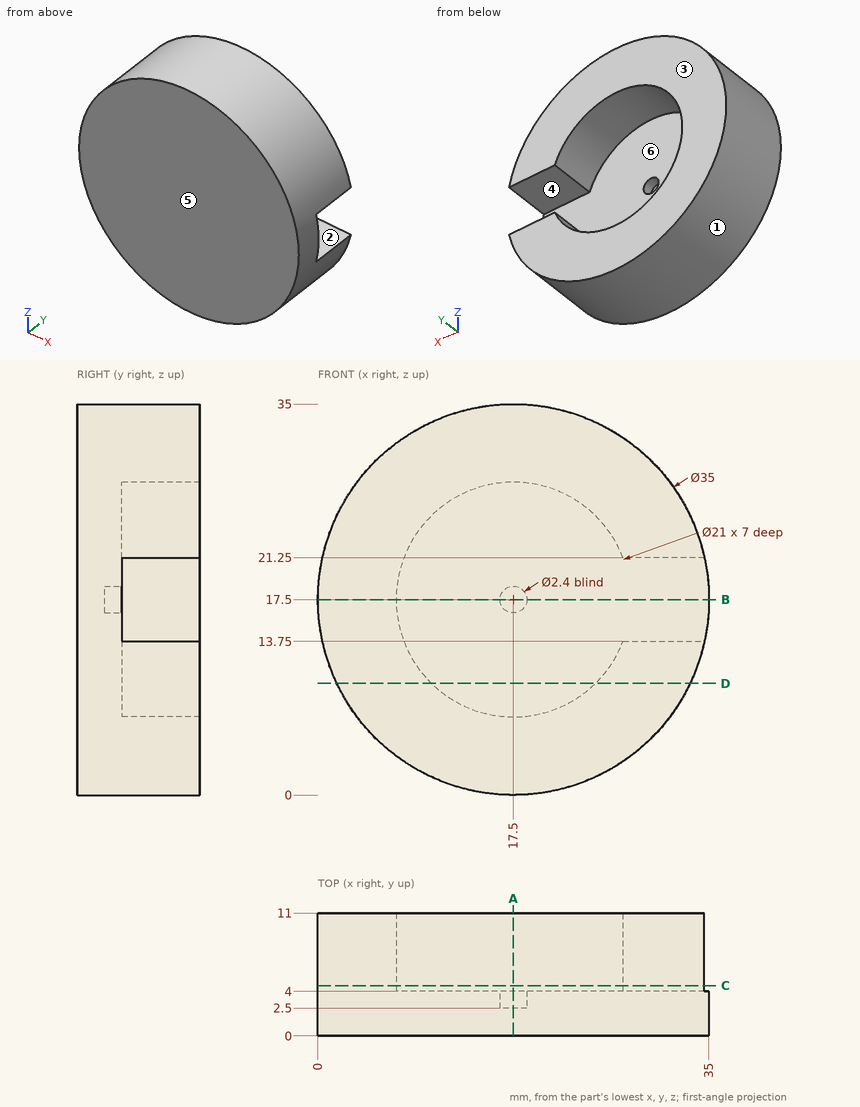
Verification items for this drawing (mm, ordinates from the low corner). A direction names the side the tool comes from. Round coordinates to 2 decimals unless told otherwise and drop trailing zeros. Order: outer loops, then holes, each group sorted by start corner. A loop starts at its lowest first (then second) coordinate and runs counter-clockwise, first axis right, second up. Notation, with made-up numbers: M 34,24 L 41,24 A24 ccw 41,63 Z; hole C 88.25,3 d3. An arc over 180 degrees is marked long. Answer in a Markdown table with one row per item. Add a question column.
Item 1: Sectioned sample at A-A, the plane x = 17.5. Enter the section's corners in (y, z).
Item 2: Material ranges on L1, parallel to Z at x = 17.5, y = 9.5; L2, parallel to Z at x = 17.5, y = 3.35; L3, parallel to Y at x = 22, z = 24.5, recorded low to high. Write a range as [from, to].
Item 3: Draft check along Z on the marked faces 1, 2, 3 and 4. Enter one of: released by +Z, released by -Z, zero draft, split by the parting line, or undercut.
Item 4: Depth check by flat-ended pin: pin 1 Ø0.7 at (x, z) = (17, 17.5) entering from +Y; pin 2 Ø5.5 at (x, y) = (31, 9) entering from -Z; pin 3 Ø4 at (y, z) = (3.5, 5.5) entering from -X. Enter the tip coordinate at first touch or a pass-through.
Item 5: Sectioned sample at D-D, the plane z = 10. Enter the section's corners in (x, y).
Item 6: Sectioned sample at B-B, the plane z = 17.5. Enter the section's corners in (x, y).
Item 7: Set-up check for the marked faces 5 and 6: record each of +Z, -Z, +X, -X, +Y, -Y from which the full face is reachable in a straight line by a thin tool's end or side.
Item 8: Sectioned sample at C-C, the plane y = 4.5. Enter the section's corners in (x, z), plus the area to 3 significant figures.
Filled in:
| question | item | result |
|---|---|---|
| 1 | outline | M 0,0 L 11,0 L 11,7 L 4,7 L 4,16.3 L 2.5,16.3 L 2.5,18.7 L 4,18.7 L 4,28 L 11,28 L 11,35 L 0,35 Z |
| 2 | L1 | z = [0, 7], [28, 35] |
| 2 | L2 | z = [0, 16.3], [18.7, 35] |
| 2 | L3 | y = [0, 4] |
| 3 | face 1 | split by the parting line |
| 3 | face 2 | undercut |
| 3 | face 3 | zero draft |
| 3 | face 4 | undercut |
| 4 | pin 1 | stops at y = 2.5 |
| 4 | pin 2 | stops at z = 3.69 |
| 4 | pin 3 | stops at x = 3.14 |
| 5 | outline | M 1.69,0 L 33.31,0 L 33.31,11 L 24.85,11 L 24.85,4 L 10.15,4 L 10.15,11 L 1.69,11 Z |
| 6 | outline | M 0,0 L 35,0 L 35,4 L 18.7,4 L 18.7,2.5 L 16.3,2.5 L 16.3,4 L 7,4 L 7,11 L 0,11 Z |
| 7 | face 5 | +Z, -Z, +X, -X, -Y |
| 7 | face 6 | +Y |
| 8 | outline | M 27.31,13.75 A10.5 cw long 27.31,21.25 L 34.59,21.25 A17.5 ccw long 34.59,13.75 Z |
| 8 | area | 563 mm² |
